Autodesk Inventor part; units mm, degrees
ref_plane "YZ Plane" through (0, 0, 0) normal (1, 0, 0) x (0, 1, 0)
ref_plane "XZ Plane" through (0, 0, 0) normal (0, 1, 0) x (-1, 0, 0)
ref_plane "XY Plane" through (0, 0, 0) normal (0, 0, 1) x (1, 0, 0)
sketch "Sketch1" plane through (0, 0, 0) normal (0, 0, 1) x (1, 0, 0)
  line L0 (-257.9687, -254) -> (257.9688, -254)
  line L1 (257.9688, -254) -> (257.9687, 254)
  line L2 (257.9687, 254) -> (-257.9688, 254)
  line L3 (-257.9688, 254) -> (-257.9687, -254)
  line L4 (-257.9687, -254) -> (257.9687, 254) construction
  line L5 (257.9688, -254) -> (-257.9688, 254) construction
  line L6 (232.5688, -228.6) -> (-232.5687, -228.6)
  line L7 (-232.5687, -228.6) -> (-232.5688, 228.6)
  line L8 (-232.5688, 228.6) -> (232.5687, 228.6)
  line L9 (232.5687, 228.6) -> (232.5688, -228.6)
  point P0 (0, 0)
  dimension "d0" = 515.9375
  dimension "d1" = 508
  dimension "d2" = 25.4
extrude "Extrusion1" add sketch "Sketch1" along normal blind 2.6568
sketch "Sketch2" plane through (0, 0, 2.6568) normal (0, 0, 1) x (1, 0, 0)
  line L0 (-257.9688, 254) -> (-257.9687, -254)
  line L1 (-257.9688, 254) -> (257.9688, 254)
  line L2 (257.9688, 254) -> (257.9688, -254)
  line L3 (257.9688, -254) -> (-257.9688, -254)
  line L4 (-257.9688, -254) -> (-257.9688, 254)
  line L5 (-253.3831, -249.4144) -> (253.3831, -249.4144)
  line L6 (253.3831, -249.4144) -> (253.3831, 249.4144)
  line L7 (253.3831, 249.4144) -> (-253.3831, 249.4144)
  line L8 (-253.3831, 249.4144) -> (-253.3831, -249.4144)
  point P0 (0, 0)
extrude "Extrusion2" add sketch "Sketch2" along normal blind 25.4
fillet "Fillet1" radius 3.175 8 edges at (-253.3831, 0, 2.6568) (0, -249.4144, 2.6568) (-253.3831, -249.4144, 15.3568) (253.3831, 0, 2.6568) (253.3831, -249.4144, 15.3568) (0, 249.4144, 2.6568) (253.3831, 249.4144, 15.3568) (-253.3831, 249.4144, 15.3568)
properties part number "rackBase"
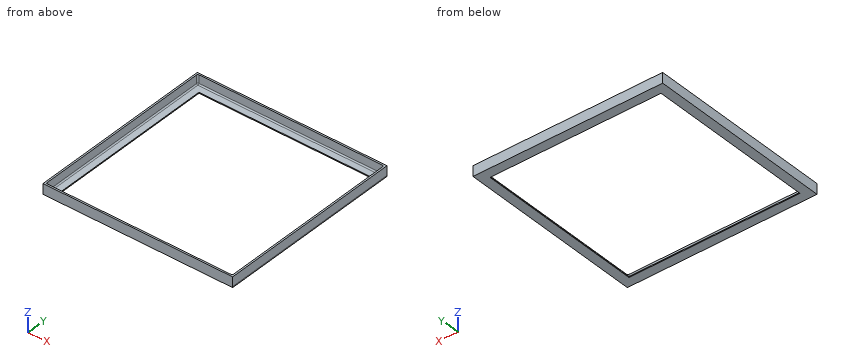
Input: part model. Units: mm. Frame: model coordinates. Coordinates: 2 decimals unless noted, no trailing zeros. Write each loop counter-clockwise with the first axis right and the second up, starting at its lowest first coordinate (ties: lowest second). Pieces come first, ordered by that corner, then holes. Notation, with made-up numbers: (26.5, 26) -> (37.5, 26) arc R13 cw to (37.5, 34) -> close; hole circle Ø7 at (-34.5, 78). An arc over 180 degrees is marked (long way). Answer as a JSON object with one key per item and string values.
1. Section A-A on x = -82. Return the cut outline in (y, z) (3 decimals), then the cut area to 3 significant figures.
Result set:
{"outline": "(-254, 0) -> (-228.6, 0) -> (-228.6, 2.657) -> (-246.239, 2.657) arc R3.175 cw to (-249.414, 5.832) -> (-249.414, 28.057) -> (-254, 28.057) -> close; (228.6, 0) -> (254, 0) -> (254, 28.057) -> (249.414, 28.057) -> (249.414, 5.832) arc R3.175 cw to (246.239, 2.657) -> (228.6, 2.657) -> close", "area": "372 mm2"}
2. Material intervals for line 1 (Y direction, x = 122, z = 7); line 2 (Y direction, x = 189, z = 2); line 3 (X direction, y = -39, z = 16.75), sorted ascending. Write a range as from..to.
Result set:
{"line 1": "y = -254..-249.41, 249.41..254", "line 2": "y = -254..-228.6, 228.6..254", "line 3": "x = -257.97..-253.38, 253.38..257.97"}
3. Section B-B on z = 23.5. Return the cut outline in (x, y) (3 decimals), then the cut area to 3 significant figures.
Result set:
{"outline": "(-257.969, -254) -> (257.969, -254) -> (257.969, 254) -> (-257.969, 254) -> close; hole (-253.383, -246.239) arc R3.175 ccw to (-250.208, -249.414) -> (250.208, -249.414) arc R3.175 ccw to (253.383, -246.239) -> (253.383, 246.239) arc R3.175 ccw to (250.208, 249.414) -> (-250.208, 249.414) arc R3.175 ccw to (-253.383, 246.239) -> close", "area": "9,320 mm2"}
